Source: CAD feature listing. Evaluate the final solid. Frame: model axes, mm. A direction names the side the tool comes from. Coordinates: 2 decimals unless noted, no trailing zeros. Write each loop counter-clockwise with the first axis right and the second up, starting at its lowest first coordinate (ties: lowest second). Pieces come first, ordered by that corner, then holes. Notation, with made-up numbers: (20.25, -5) -> (71.25, -5) arc R20 ccw to (71.25, 14) -> close; hole circle Ø4 at (69, -12.75). An arc over 180 degrees is marked (long way). One line per item, written item: value. Start each with the question number.
1. Access query for faces 1 (the flat face through (2.8, -0.8, 4.572)), 2 (the flat face through (-2.65, -0.56, 2.25)). Directions: +Z, -Z, +X, -X, +Y, -Y. A direction counts if a zero-diameter tool reaches every point of the face in a straight line with its end or side. Return the directions, or none.
2. Section query C-C, the plane z = 7. State how many separate pieces and enclosed holes the cut face has, and give its area (3 significant figures).
3. Mould query, pull axis X, two halves, no side actions, for faces 3 (the cylindrical face through (-1.38, -6.2, 10.12)), 4 (the flat face through (-5, 5, 7.62)), 5 (the flat face through (2.65, 0.56, 2.25)). Classes: released by +X, released by -X, zero draft, split by the parting line, or undercut.
4. Section query A-A, the plane x = 12.7. Output: boundary loops of the cut face in (y, z), and give its area (3 significant figures).
5. Line query: line 1 (Y direction, x = 0, z = 9.25) (3 decimals); line 2 (Y direction, x = 12.7, z = 5.5); line 3 (Z direction, x = -7, y = 16). Output: solid intervals per line, ascending.
6. First-contact query: P1, Ø5, axis at y = -9, z = 5.5, coming from the -X side; P2, Ø2.5, axis at x = -12.7, y = 0, coming from the +Z side; P3, Ø5.5, axis at x = 0, y = 0, coming from the +Z side; P4, Ø1, axis at y = 11, z = 8, coming from the -X side. Flat tips, straight axial feed; report the tip coordinate or a pass-through.
from build123d import *

# Parameters (mm, degrees)
F0_R     = 6.35
F0_R_2   = 3.175
F1_DEPTH = 12.7
F2_R     = 19.05
F2_R_2   = 6.35
F3_DEPTH = 7.62
F5_DEPTH = 4.572
F7_D     = 3.175


with BuildPart() as f1:
    # F0 (on Top) → F1 (new body)
    with BuildSketch(Plane.XY):
        Circle(F0_R)
        Circle(F0_R_2, mode=Mode.SUBTRACT)
    extrude(amount=F1_DEPTH)

    # F2 (on Top) → F3 (join)
    with BuildSketch(Plane.XY):
        Circle(F2_R)
        Circle(F2_R_2, mode=Mode.SUBTRACT)
    extrude(amount=F3_DEPTH)

    # F4 (on Top) → F5 (join)
    with BuildSketch(Plane.XY):
        Polygon((-0.803219, 3.429), (0, 2.286), (0, 3.429), align=None)
        Polygon((0, 3.429), (0, 2.286), (0.803219, 3.429), align=None)
        Polygon((1.365698, 3.246239), (1.343677, 1.849413), (2.015516, 2.774119), align=None)
        Polygon((2.015516, 2.774119), (1.343677, 1.849413), (2.665333, 2.301999), align=None)
        Polygon((3.012965, 1.823525), (2.174115, 0.706413), (3.261173, 1.059619), align=None)
        Polygon((3.261173, 1.059619), (2.174115, 0.706413), (3.509381, 0.295713), align=None)
        Polygon((0, -2.286), (-0.803219, -3.429), (0, -3.429), align=None)
        Polygon((0.803219, -3.429), (0, -2.286), (0, -3.429), align=None)
        Polygon((1.365698, -3.246239), (2.015516, -2.774119), (1.343677, -1.849413), align=None)
        Polygon((1.343677, -1.849413), (2.015516, -2.774119), (2.665333, -2.301999), align=None)
        Polygon((3.012965, -1.823525), (3.261173, -1.059619), (2.174115, -0.706413), align=None)
        Polygon((2.174115, -0.706413), (3.261173, -1.059619), (3.509381, -0.295713), align=None)
        Polygon((-2.665333, 2.301999), (-1.343677, 1.849413), (-2.015516, 2.774119), align=None)
        Polygon((-2.015516, 2.774119), (-1.343677, 1.849413), (-1.365698, 3.246239), align=None)
        Polygon((-3.012965, 1.823525), (-3.261173, 1.059619), (-2.174115, 0.706413), align=None)
        Polygon((-2.174115, 0.706413), (-3.261173, 1.059619), (-3.509381, 0.295713), align=None)
        Polygon((-3.261173, -1.059619), (-2.174115, -0.706413), (-3.509381, -0.295713), align=None)
        Polygon((-3.012965, -1.823525), (-2.174115, -0.706413), (-3.261173, -1.059619), align=None)
        Polygon((-2.015516, -2.774119), (-1.343677, -1.849413), (-2.665333, -2.301999), align=None)
        Polygon((-1.365698, -3.246239), (-1.343677, -1.849413), (-2.015516, -2.774119), align=None)
    extrude(amount=F5_DEPTH)

    # F7 (through all)
    with Locations(Plane.XY.offset(7.62)):
        with Locations((0, -12.7), (-12.7, 0), (0, 12.7), (12.7, 0)):
            Hole(F7_D / 2)


solid = f1.part
Computed values:
1. face 1: +Z
1. face 2: +Z, -Z
2. separate pieces: 1
2. enclosed holes: 5
2. area: 1,080 mm²
3. face 3: split by the parting line
3. face 4: zero draft
3. face 5: undercut
4. outline: (-14.2, 0) -> (-1.59, 0) -> (-1.59, 7.62) -> (-14.2, 7.62) -> close; (1.59, 0) -> (14.2, 0) -> (14.2, 7.62) -> (1.59, 7.62) -> close
4. area: 192 mm²
5. line 1: y = -6.35 to -3.175, 3.175 to 6.35
5. line 2: y = -14.2 to -1.59, 1.59 to 14.2
5. line 3: z = 0 to 7.62
6. P1: stops at x = -17.91
6. P2: passes through
6. P3: stops at z = 4.57
6. P4: stops at x = -15.78
